from build123d import *

# Parameters (mm, degrees)
F0_R      = 65.437534
F1_DEPTH  = 25.4
F2_R      = 51.719022
F3_DEPTH  = 12.929184
F4_R      = 51.719022
F4_R_2    = 2.585787
F4_R_3    = 65.262229
F5_DEPTH  = 25.4
F6_R      = 47.073504
F7_DEPTH  = 61.468
F8_R      = 50.226774
F8_R_2    = 2.585787
F9_DEPTH  = 74.93
F11_W     = 9.235289
F11_H     = 11.885514
F10_R     = 47.073504
F12_DEPTH = 1.524
F13_W     = 3.887014
F13_H     = 3.9601
F14_DEPTH = 53.34


with BuildPart() as f1:
    # F0 (on Top) → F1 (new body)
    with BuildSketch(Plane.XY):
        Circle(F0_R)
    extrude(amount=F1_DEPTH)

    # F2 (on face) → F3 (join)
    with BuildSketch(Plane.XY.offset(25.4)):
        Circle(F2_R)
    extrude(amount=F3_DEPTH)

    # F4 (on face) → F5 (join)
    with BuildSketch(Plane.XY.offset(38.329184)):
        Circle(F4_R)
        Circle(F4_R_2, mode=Mode.SUBTRACT)
        Circle(F4_R_3)
        Circle(F4_R_2, mode=Mode.SUBTRACT)
    extrude(amount=F5_DEPTH)

    # F6 (on face) → F7 (join)
    with BuildSketch(Plane(origin=(0, 0, 0), x_dir=(1, 0, 0), z_dir=(0, 0, -1))):
        Circle(F6_R)
    extrude(amount=F7_DEPTH)

    # F8 (on face) → F9 (join)
    with BuildSketch(Plane.XY.offset(63.729184)):
        with Locations((-2.585787, 0)):
            Circle(F8_R)
        Circle(F8_R_2, mode=Mode.SUBTRACT)
    extrude(amount=F9_DEPTH)

    # F11 (on face) + F10 (on face) → F12 (join)
    with BuildSketch(Plane(origin=(0, 0, -61.468), x_dir=(1, 0, 0), z_dir=(0, 0, -1))):
        with Locations((0.111258, -0.588183)):
            Rectangle(F11_W, F11_H)
    with BuildSketch(Plane(origin=(0, 0, -61.468), x_dir=(1, 0, 0), z_dir=(0, 0, -1))):
        Circle(F10_R)
    extrude(amount=-F12_DEPTH)

    # F13 (on face) → F14 (join)
    with BuildSketch(Plane(origin=(0, 0, -61.468), x_dir=(1, 0, 0), z_dir=(0, 0, -1))):
        with Locations((-0.249897, -0.261744)):
            Rectangle(F13_W, F13_H)
    extrude(amount=F14_DEPTH)


solid = f1.part
Work out the finished part from the listing and answer in its coordinate system (mm). A direction names the side the tool comes from. Give positions to 0.01 mm unless a question says otherwise; leave off trailing zeros. Loops run counter-clockwise (first coordinate to the right, second up) from the corner with the lowest first, then second, coordinate; pieces in that order, holes last. Notation, with made-up numbers: M -34,50.25 L 3,50.25 A20 ccw 3,61.25 Z; hole C 86,11 d4. An arc over 180 degrees is marked long. Use CSV: the item, a comma, the result in double quotes.
1) Find section B-B on y = -41. Write down the section's boundary in (x, z), plus the area to 3 significant figures.
Answer:
outline,"M -51,0 L -23.13,0 L -23.13,-61.47 L 23.13,-61.47 L 23.13,0 L 51,0 L 51,25.4 L 31.53,25.4 L 31.53,38.33 L 50.78,38.33 L 50.78,63.73 L 26.43,63.73 L 26.43,138.66 L -31.6,138.66 L -31.6,63.73 L -50.78,63.73 L -50.78,38.33 L -31.53,38.33 L -31.53,25.4 L -51,25.4 Z"
area,"13,200 mm^2"
2) Determine the mould class of faces 1 (the cylindrical face through (-0.561, -2.524, 87.792)), 2 (the flat face through (48, -5, 63.729)), 3 (the flat face through (0, 0, 38.329)), 4 (the cylindrical face through (49.331, 15.535, 31.774)) for opening direction Y: released by +Y, released by -Y, zero draft, split by the parting line, or undercut.
Answer:
face 1,"undercut"
face 2,"zero draft"
face 3,"undercut"
face 4,"split by the parting line"
3) Given P1, Ø1.2, axis at y = 0, z = -83, coming from the +X side; P2, Ø6, axis at x = 0, y = 0, coming from the +Z side; P3, Ø12, axis at y = 8, z = 59.5, coming from the +X side; P4, Ø4.5, axis at x = -1, z = -97, coming from the -Y side, each flat-ended and moving along its own axis, determine where each tip first touches the part or whether it passes through.
Answer:
P1,"x = 1.69"
P2,"z = 138.66"
P3,"x = 65.23"
P4,"y = -1.72"
4) Find section A-A on z = -28. Write down the section's boundary in (x, y), plus the area to 3 significant figures.
Answer:
outline,"C 0,0 d94.15"
area,"6,960 mm^2"
5) Which of the six approach directions +Z, -Z, +X, -X, +Y, -Y give full straight-line access (tool end or side, diameter ignored) to faces 5 (the cylindrical face through (-9.12, 49.8, 100.67)), 6 (the flat face through (-20, 49, 38.329)), 7 (the flat face through (-15, 45, 0))?
Answer:
face 5,"+Z"
face 6,"none"
face 7,"-Z"
6) Consider L1, parallel to Z at x = -8.5, y = 56.5; L2, parallel to Z at x = -13, y = 46; L3, parallel to Y at x = -2, z = -45. Determine where each line is inside the solid, lowest interval first.
Answer:
L1,"0 to 25.4, 38.33 to 63.73"
L2,"0 to 138.66"
L3,"-47.03 to 47.03"
7) Find section D-D on x = -34. Write down the section's boundary in (y, z).
Answer:
outline,"M -55.91,0 L -32.56,0 L -32.56,-61.47 L 32.56,-61.47 L 32.56,0 L 55.91,0 L 55.91,25.4 L 38.97,25.4 L 38.97,38.33 L 55.71,38.33 L 55.71,63.73 L 39.19,63.73 L 39.19,138.66 L -39.19,138.66 L -39.19,63.73 L -55.71,63.73 L -55.71,38.33 L -38.97,38.33 L -38.97,25.4 L -55.91,25.4 Z"
8) Find section C-C on z = 88.5. Write down the section's boundary in (x, y).
Answer:
outline,"C -2.59,0 d100.45; hole C 0,0 d5.17"
